Model file for the job. Use its own axes, mm. A direction names the side the tool comes from. Give positions to 0.01 mm unless a question says otherwise; leave off trailing zeros. Loops run counter-clockwise (first coordinate to the right, second up) from the corner with the lowest first, then second, coordinate; pieces in that order, holes last. Notation, with made-up numbers: (43.25, -31) - (76.25, -31) arc R14 cw to (76.25, -10) - close; hole circle Ø8 at (-32, 82). An arc over 180 degrees is marked (long way). Use a Markdown table: item, result.
Autodesk Inventor part; units mm, degrees
ref_plane "YZ Plane" through (0, 0, 0) normal (1, 0, 0) x (0, 1, 0)
ref_plane "XZ Plane" through (0, 0, 0) normal (0, 1, 0) x (-1, 0, 0)
ref_plane "XY Plane" through (0, 0, 0) normal (0, 0, 1) x (1, 0, 0)
sketch "Sketch1" plane through (0, 0, 0) normal (0, 1, 0) x (-1, 0, 0)
  line L0 (-33.5, 26) -> (33.5, 26)
  line L1 (33.5, 26) -> (33.5, -26)
  line L2 (-33.5, -26) -> (-33.5, 26)
  line L3 (-33.5, 26) -> (33.5, -26) construction
  line L4 (33.5, 26) -> (-33.5, -26) construction
  line L5 (33.5, 0) -> (28, 0)
  line L6 (28, 7.5) -> (28, -7.5)
  line L7 (30.5, 7.5) -> (25.5, 7.5)
  line L8 (25.5, 7.5) -> (25.5, 17.5)
  line L9 (25.5, 17.5) -> (30.5, 17.5)
  line L10 (30.5, 17.5) -> (30.5, 7.5)
  line L11 (30.5, -7.5) -> (25.5, -7.5)
  line L12 (25.5, -7.5) -> (25.5, -17.5)
  line L13 (25.5, -17.5) -> (30.5, -17.5)
  line L14 (30.5, -17.5) -> (30.5, -7.5)
  line L15 (22.5, -23) -> (-27.5, -23)
  line L16 (-27.5, -23) -> (-27.5, -4)
  line L17 (-27.5, -4) -> (22.5, -4)
  line L18 (22.5, -4) -> (22.5, -23)
  line L19 (12.5, 23) -> (-30.5, 23)
  line L20 (-30.5, 23) -> (-30.5, 2)
  line L21 (-30.5, 2) -> (12.5, 2)
  line L22 (12.5, 2) -> (12.5, 23)
  line L23 (25.5, 12.5) -> (12.5, 12.5)
  line L24 (-33.5, -26) -> (33.5, -26)
  line L25 (12.5, 16.5) -> (25.5, 16.5)
  line L26 (12.5, 8.5) -> (25.5, 8.5)
  line L27 (25.5, 16.5) -> (22.5, 16.5)
  line L28 (22.5, 16.5) -> (22.5, 13.5)
  line L29 (22.5, 13.5) -> (25.5, 13.5)
  line L30 (22.5, 13.5) -> (22.5, 11.5)
  line L31 (22.5, 11.5) -> (22.5, 8.5)
  line L32 (22.5, 11.5) -> (25.5, 11.5)
  line L33 (24.2677, 11.5) -> (24.2677, 13.5)
  point P0 (0, 0)
  point P1 (24.2677, 12.5)
  dimension "d3" = 15
  dimension "d5" = 10
  dimension "d6" = 5
  dimension "d11" = 50
  dimension "d12" = 3
  dimension "d13" = 43
  dimension "d14" = 13
  dimension "d22" = 19
  dimension "d23" = 21
  dimension "d26" = 3
  dimension "d27" = 3
  dimension "d28" = 3
  dimension "d29" = 3
  dimension "d30" = 6
  dimension "d31" = 67
  dimension "d32" = 52
  dimension "d33" = 8
  dimension "d34" = 3
  dimension "d35" = 2
extrude "Extrusion1" add sketch "Sketch1" along normal blind 16 contours L0 L1 L24 L2 | L26 L31 L32 L8 | L32 L33 L23 L8 | L26 L22 L23 L30 L31 | L8 L29 L28 L25 | L23 L33 L29 L8 | L32 L30 L23 L33 | L28 L30 L23 L22 L25 | L23 L30 L29 L33
sketch "Sketch2" plane through (0, 16, 0) normal (0, 1, 0) x (1, 0, 0)
  line L0 (-12.5, -16.5) -> (-25.5, -16.5)
  line L1 (-12.5, -8.5) -> (-25.5, -8.5)
  line L2 (-22.5, -11.5) -> (-22.5, -8.5)
  line L3 (-22.5, -16.5) -> (-22.5, -13.5)
  line L4 (-22.5, -11.5) -> (-25.5, -11.5)
  line L5 (-22.5, -13.5) -> (-25.5, -13.5)
  line L6 (-25.5, -7.5) -> (-25.5, -17.5)
  line L7 (-12.5, -2) -> (-12.5, -23)
  line L8 (-22.5, -13.5) -> (-22.5, -11.5)
  point P0 (0, 0)
extrude "Extrusion4" cut sketch "Sketch2" against normal blind 13 contours L0 L3 L8 L2 L1 L7
extrude "Extrusion5" cut sketch "Sketch2" against normal blind 10 contours L5 L6 L4 L8
extrude "Extrusion6" add sketch "Sketch1" against normal blind 3 contours L0 L1 L24 L2 | L26 L31 L32 L8 | L32 L33 L23 L8 | L26 L22 L23 L30 L31 | L8 L29 L28 L25 | L23 L33 L29 L8 | L32 L30 L23 L33 | L22 L21 L20 L19 | L28 L30 L23 L22 L25 | L23 L30 L29 L33 | L15 L16 L17 L18
properties part number "Bund"
(1) Slice it at B-B, the plane y = 1. Write the cut outline in (x, z), plus the area to 3 significant figures.
Computed:
| item | result |
|---|---|
| outline | (-33.5, -26) - (33.5, -26) - (33.5, 26) - (-33.5, 26) - close; hole (-30.5, -17.5) - (-25.5, -17.5) - (-25.5, -7.5) - (-30.5, -7.5) - close; hole (-30.5, 7.5) - (-25.5, 7.5) - (-25.5, 17.5) - (-30.5, 17.5) - close; hole (-22.5, -23) - (27.5, -23) - (27.5, -4) - (-22.5, -4) - close; hole (-12.5, 2) - (30.5, 2) - (30.5, 23) - (-12.5, 23) - close |
| area | 1,530 mm² |
(2) Slice it at C-C, the plane x = 8. Write the cut outline in (y, z).
Computed:
| item | result |
|---|---|
| outline | (-3, -26) - (16, -26) - (16, -23) - (0, -23) - (0, -4) - (16, -4) - (16, 2) - (0, 2) - (0, 23) - (16, 23) - (16, 26) - (-3, 26) - close |
(3) Pin check, flat tips, straight feed: P1, Ø0.6, axis at x = -24.5, z = 12.5, coming from the +Y side; P2, Ø17, axis at x = 16, z = 16.5, coming from the +Y side; P3, Ø9.5, axis at x = -6, z = -16.5, coming from the +Y side. Stop position of each tip, or through.
Computed:
| item | result |
|---|---|
| P1 | y = 6 |
| P2 | y = 16 |
| P3 | y = 0 |
(4) Slice it at A-A, the plane z = 15.5. Write the cut outline in (x, y).
Computed:
| item | result |
|---|---|
| outline | (-33.5, -3) - (-30.5, -3) - (-30.5, 16) - (-33.5, 16) - close; (-25.5, -3) - (33.5, -3) - (33.5, 16) - (30.5, 16) - (30.5, 0) - (-12.5, 0) - (-12.5, 3) - (-22.5, 3) - (-22.5, 16) - (-25.5, 16) - close |
(5) Slice it at D-D, the plane z = -21.5. Write the cut outline in (x, y).
Computed:
| item | result |
|---|---|
| outline | (-33.5, -3) - (33.5, -3) - (33.5, 16) - (27.5, 16) - (27.5, 0) - (-22.5, 0) - (-22.5, 16) - (-33.5, 16) - close |
(6) Mould opens along X. For faces 1 (the flat face through (-33.5, 6, 0)), 2 (the flat face through (33.5, 6, 0)), 3 (the flat face through (-25.5, 6, -12)), 4 (the flat face through (0, 6, -26)) say: pulls with the +X half, pulls with the -X half, needs draft (parallel to the pull), parting line crosses it, or undercut.
Computed:
| item | result |
|---|---|
| face 1 | pulls with the -X half |
| face 2 | pulls with the +X half |
| face 3 | undercut |
| face 4 | needs draft |
(7) 3-axis set-ups, long thin cutter, end or side, ignore diameter. For faces 5 (the flat face through (-24, 6, 12)), 6 (the flat face through (-30.5, 6, 13)): which of +Z, -Z, +X, -X, +Y, -Y reach the whole face in a straight line?
Computed:
| item | result |
|---|---|
| face 5 | +Y |
| face 6 | +Y, -Y |
(8) Drill centre lines: probe 1 along Z at (x, y) = (1, 8.75); probe 2 along Z at (x, y) = (-27, 14.75); probe 3 along X at (y, z) = (4.25, -14). Where is each one in solid material? Low to high. Write a range as [from, to].
Computed:
| item | result |
|---|---|
| probe 1 | [-26, -23], [-4, 2], [23, 26] |
| probe 2 | [-26, -17.5], [-7.5, 7.5], [17.5, 26] |
| probe 3 | [-33.5, -30.5], [-25.5, -22.5], [27.5, 33.5] |
